from build123d import *

# Parameters (mm, degrees)
SKETCH1_R           = 11
BOSS_EXTRUDE1_DEPTH = 25.4
SKETCH13_W          = 60
SKETCH13_H          = 60
BOSS_EXTRUDE5_DEPTH = 20
FACE_1_R            = 9.25
CUT_EXTRUDE1_DEPTH  = 20
FACE_3_R            = 9.25
CUT_EXTRUDE2_DEPTH  = 20
CUT_EXTRUDE3_START  = -20
FACE_2_R            = 9.25
CUT_EXTRUDE3_DEPTH  = 20


with BuildPart() as part:
    # Sketch1 → Boss-Extrude1 (new body)
    with BuildSketch(Plane(origin=(0, 0, 0), x_dir=(1, 0, 0), z_dir=(0, 1, 0))):
        with Locations(Location((0, 0, 0), (0, 0, 270))):
            Circle(SKETCH1_R)
    extrude(amount=BOSS_EXTRUDE1_DEPTH)

    # Sketch13 → Boss-Extrude5 (add)
    with BuildSketch(Plane(origin=(0, 25.4, 0), x_dir=(1, 0, 0), z_dir=(0, 1, 0))):
        Rectangle(SKETCH13_W, SKETCH13_H)
    extrude(amount=BOSS_EXTRUDE5_DEPTH)

    # Face 1 → Cut-Extrude1 (cut)
    with BuildSketch(Plane.XY.offset(30)):
        with Locations((0, 35.4)):
            Circle(FACE_1_R)
    extrude(amount=-CUT_EXTRUDE1_DEPTH, mode=Mode.SUBTRACT)

    # Face 3 → Cut-Extrude2 (cut)
    with BuildSketch(Plane.ZY.offset(30)):
        with Locations((0, 35.4)):
            Circle(FACE_3_R)
    extrude(amount=-CUT_EXTRUDE2_DEPTH, mode=Mode.SUBTRACT)

    # Face 2 → Cut-Extrude3 (cut)
    with BuildSketch(Plane(origin=(30, 0, 0), x_dir=(0, 0, -1), z_dir=(1, 0, 0)).offset(CUT_EXTRUDE3_START)):
        with Locations(Location((0, 35.4, 0), (0, 0, 180))):
            Circle(FACE_2_R)
    extrude(amount=CUT_EXTRUDE3_DEPTH, mode=Mode.SUBTRACT)


solid = part.part
Design review of the part built by this model. Coordinates are the model's own, in mm. A direction names the side the tool comes from. Coordinates: 2 decimals unless noted, no trailing zeros. Order: outer loops, then holes, each group sorted by start corner. A loop starts at its lowest first (then second) coordinate and runs counter-clockwise, first axis right, second up. Notation, with made-up numbers: (80, 1.5) -> (125, 1.5) arc R6 cw to (125, 5.5) -> close; hole circle Ø11 at (77.5, 45.25). An arc over 180 degrees is marked (long way). Use one line per item in the form item = value. Start each with the question number.
(1) Add section C-C on y = 35.4. State the section outline as (x, z) points.
(2) Add section A-A on z = 0. State the section outline as (x, y) points.
(3) For probe 1 along Z at (x, y) = (16, 35); probe 2 along Y at (x, z) = (-26, 0); probe 3 along Y at (x, z) = (6, -21.5), list the stretches that pass through material, from the lowest coordinate up.
(4) The part is to be moulded in two halves that separate along Y. For faces 1 (the flat face through (0, 0, 0)), 2 (the flat face through (0, 36, 10)), 3 (the flat face through (0, 45.4, 0)), say which applies: +Y half, -Y half, draft (parallel to the pull), parting line (faces both ways), or undercut.
(5) Add section D-D on z = 15. State the section outline as (x, y) points, plus the area to 3 significant figures.
(6) Add section B-B on x = -20.5. State the section outline as (y, z) points.
(7) Insertion check: pin 1 (6 mm diameter, centred on x = 13, z = -16.5, fed in from -Y); pin 2 (1.5 mm diameter, centred on x = 1, y = 21, fed in from -Z); pin 3 (5 mm diameter, centred on y = 35, z = -4.5, fed in from -X). Each pin has a flat end and moves straight along its axis. Give the tip position at first contact, or say it passes through.
(8) For faces 4 (the cylindrical face through (-1.2, 44.57, 20.14)), 5 (the cylindrical face through (-20.14, 44.57, -1.2)), 6 (the flat face through (10, 35, 0)), 7 (the flat face through (-30, 42, 7)), 8 (the flat face through (-14, 25.4, 0)), list the 3-axis set-ups (+Z, -Z, +X, -X, +Y, -Y) from which the entire face can be reached by the end or side of a thin tool; tool diameter is ignored.
Answer block:
q1.outline = (-30, -30) -> (30, -30) -> (30, -9.25) -> (10, -9.25) -> (10, 9.25) -> (30, 9.25) -> (30, 30) -> (9.25, 30) -> (9.25, 10) -> (-9.25, 10) -> (-9.25, 30) -> (-30, 30) -> (-30, 9.25) -> (-10, 9.25) -> (-10, -9.25) -> (-30, -9.25) -> close
q2.outline = (-30, 25.4) -> (-11, 25.4) -> (-11, 0) -> (11, 0) -> (11, 25.4) -> (30, 25.4) -> (30, 26.15) -> (10, 26.15) -> (10, 44.65) -> (30, 44.65) -> (30, 45.4) -> (-30, 45.4) -> (-30, 44.65) -> (-10, 44.65) -> (-10, 26.15) -> (-30, 26.15) -> close
q3.probe_1 = -30 to -9.24, 9.24 to 30
q3.probe_2 = 25.4 to 26.15, 44.65 to 45.4
q3.probe_3 = 25.4 to 45.4
q4.face_1 = -Y half
q4.face_2 = undercut
q4.face_3 = +Y half
q5.outline = (-30, 25.4) -> (30, 25.4) -> (30, 45.4) -> (-30, 45.4) -> close; hole circle Ø18.5 at (0, 35.4)
q5.area = 931 mm²
q6.outline = (25.4, -30) -> (45.4, -30) -> (45.4, 30) -> (25.4, 30) -> close; hole circle Ø18.5 at (35.4, 0)
q7.pin_1 = 25.4
q7.pin_2 = -11
q7.pin_3 = -10
q8.face_4 = +Z
q8.face_5 = -X
q8.face_6 = +X
q8.face_7 = +Z, -Z, -X, +Y, -Y
q8.face_8 = -Y
